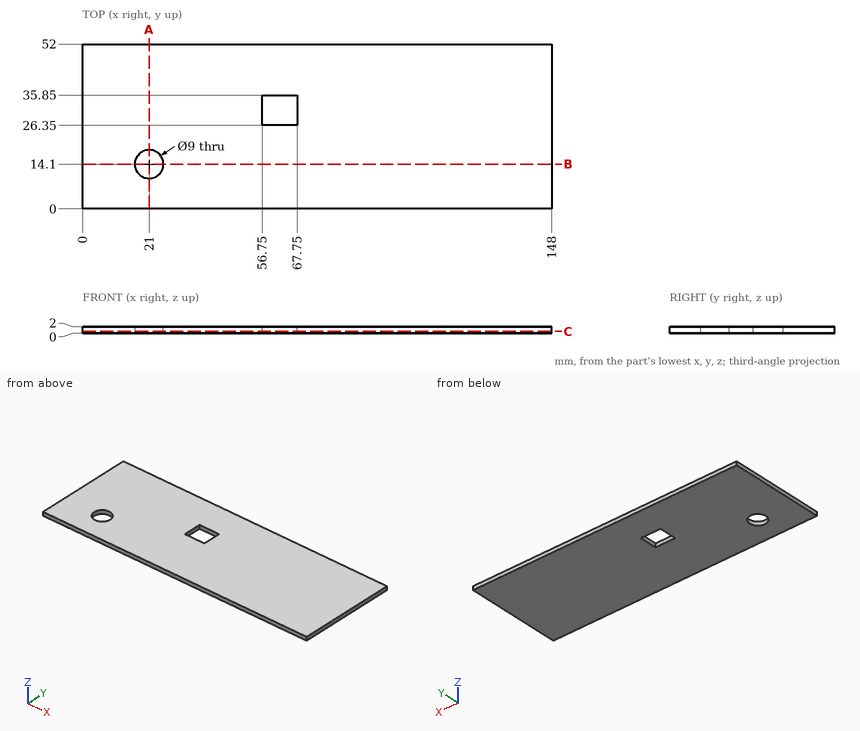
Here's the drawing with two shaded views (mm, measured from the low corner). I have some questions. Give positions to 0.01 mm unless a question says otherwise; leave off trailing zeros. Loops run counter-clockwise (first coordinate to the right, second up) from the corner with the lowest first, then second, coordinate; pieces in that order, holes last. Notation, with made-up numbers: (-28.75, 0.25) - (-9.75, 0.25) arc R28 cw to (-9.75, 23.25) - close; hole circle Ø11 at (14, 52). An arc over 180 degrees is marked (long way). One line per item, written item: value.
(1) If we section it at B-B, the plane y = 14.1: List the corners of the cut face in (x, z) for me.
Verdict:
outline: (0, 0) - (16.5, 0) - (16.5, 2) - (0, 2) - close; (25.5, 0) - (148, 0) - (148, 2) - (25.5, 2) - close
(2) If we section it at C-C, the plane z = 0.55: List the corners of the cut face in (x, y) for me, plus the area to 3 significant figures.
Verdict:
outline: (0, 0) - (148, 0) - (148, 52) - (0, 52) - close; hole circle Ø9 at (21, 14.1); hole (56.75, 26.35) - (67.75, 26.35) - (67.75, 35.85) - (56.75, 35.85) - close
area: 7,530 mm^2
(3) If we section it at A-A, the plane x = 21: List the corners of the cut face in (y, z) for me.
Verdict:
outline: (0, 0) - (9.6, 0) - (9.6, 2) - (0, 2) - close; (18.6, 0) - (52, 0) - (52, 2) - (18.6, 2) - close
(4) I need wall thicknesses on line 1 along Y through (x, z) = (21, 1.45); line 2 along X through (y, z) = (31, 1.9); line 3 along Y through (x, z) = (63, 1.7). Which ranges of each line are inside material? Lowest first, please.
Verdict:
line 1: 0 to 9.6, 18.6 to 52
line 2: 0 to 56.75, 67.75 to 148
line 3: 0 to 26.35, 35.85 to 52
